Can you work these out from the drawing? Everything is in mm from the part's minimum corner. A direction names the side the tool comes from. Round coordinates to 2 decimals unless told otherwise and drop trailing zeros. Loops run counter-clockwise (first coordinate to the right, second up) from the corner with the lowest first, then second, coordinate; pieces in that order, holes last. Notation, with made-up numbers: (39, -27.5) -> (80, -27.5) arc R22 cw to (80, -6.5) -> close; hole circle Ø5 at (37, 69.5). An arc over 180 degrees is marked (long way). One line per item, written item: value.
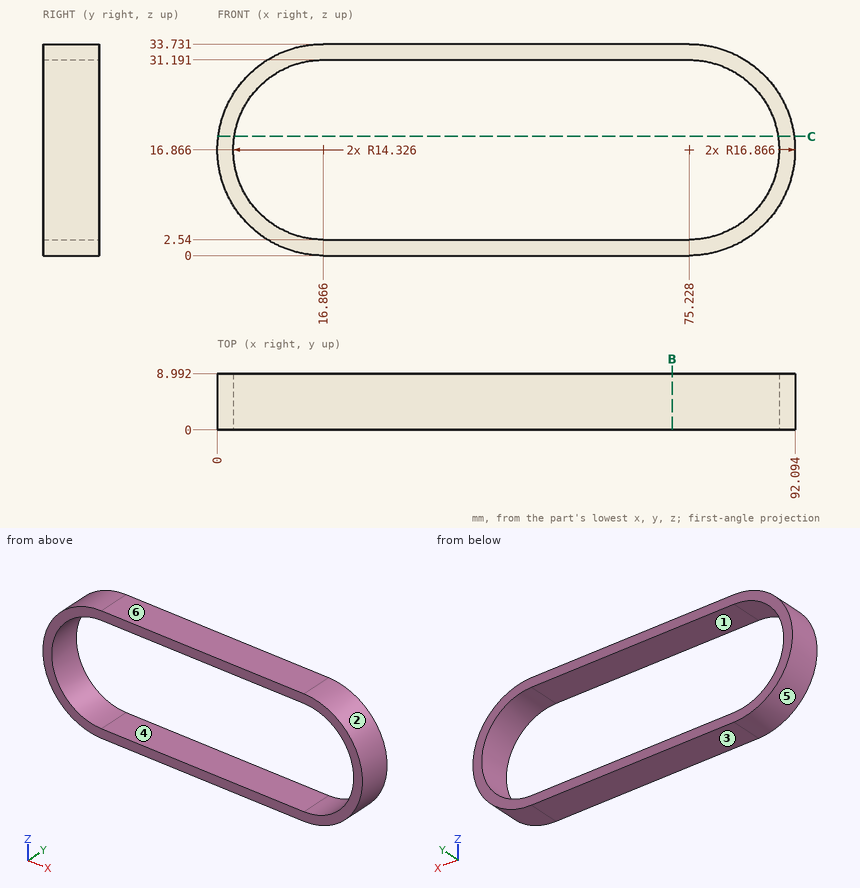
Item 1: If we mould it in two halves opening along Z, with no side actions, what happens to the marked faces 3, 4, 5 and 6? For each: released by +Z, released by -Z, zero draft, split by the parting line, or undercut.
Output:
face 3: released by -Z
face 4: undercut
face 5: split by the parting line
face 6: released by +Z
Item 2: For the marked faces 1 and 2, which set-ups out of +Z, -Z, +X, -X, +Y, -Y let a thin tool reach every point of the face, with its end or its side?
Output:
face 1: +Y, -Y
face 2: +X, +Y, -Y
Item 3: I need wall thicknesses on line 1 (X direction, y = 1, z = 17); line 2 (Z direction, x = 72, y = 2.25); line 3 (X direction, y = 2, z = 7) (1 decimal). Which ranges of each line are inside material? Lowest first, please. Write a range as from..to.
Output:
line 1: x = 0..2.54, 89.55..92.09
line 2: z = 0..2.54, 31.19..33.73
line 3: x = 3.2..6.5, 85.6..88.9
Item 4: If we section it at C-C on z = 19: List the corners of the cut face in (x, y) for me (1 decimal).
Output:
outline: (0.1, 0) -> (2.7, 0) -> (2.7, 9) -> (0.1, 9) -> close; (89.4, 0) -> (92, 0) -> (92, 9) -> (89.4, 9) -> close
Item 5: Will these pins go through, and if not, where does the flat tip stop? pin 1 Ø10 at (x, z) = (15, 21.5) entering from -Y; pin 2 Ø3 at (x, y) = (79, 1) entering from +Z.
Output:
pin 1: passes through
pin 2: stops at z = 33.58
Item 6: If we section it at B-B on x = 72.5: List the corners of the cut face in (y, z) for me.
Output:
outline: (0, 0) -> (8.99, 0) -> (8.99, 2.54) -> (0, 2.54) -> close; (0, 31.19) -> (8.99, 31.19) -> (8.99, 33.73) -> (0, 33.73) -> close
